Answer from the drawing. Dimensions are ordinates in mm from the lowest x, y and z of the part. A direction names the side the tool comes from. Coordinates: 2 decimals unless noted, no trailing zeros. Order: outer loops, then holes, each group sorted by start corner. A loop starts at its lowest first (then second) coordinate and runs counter-clockwise, first axis right, second up.
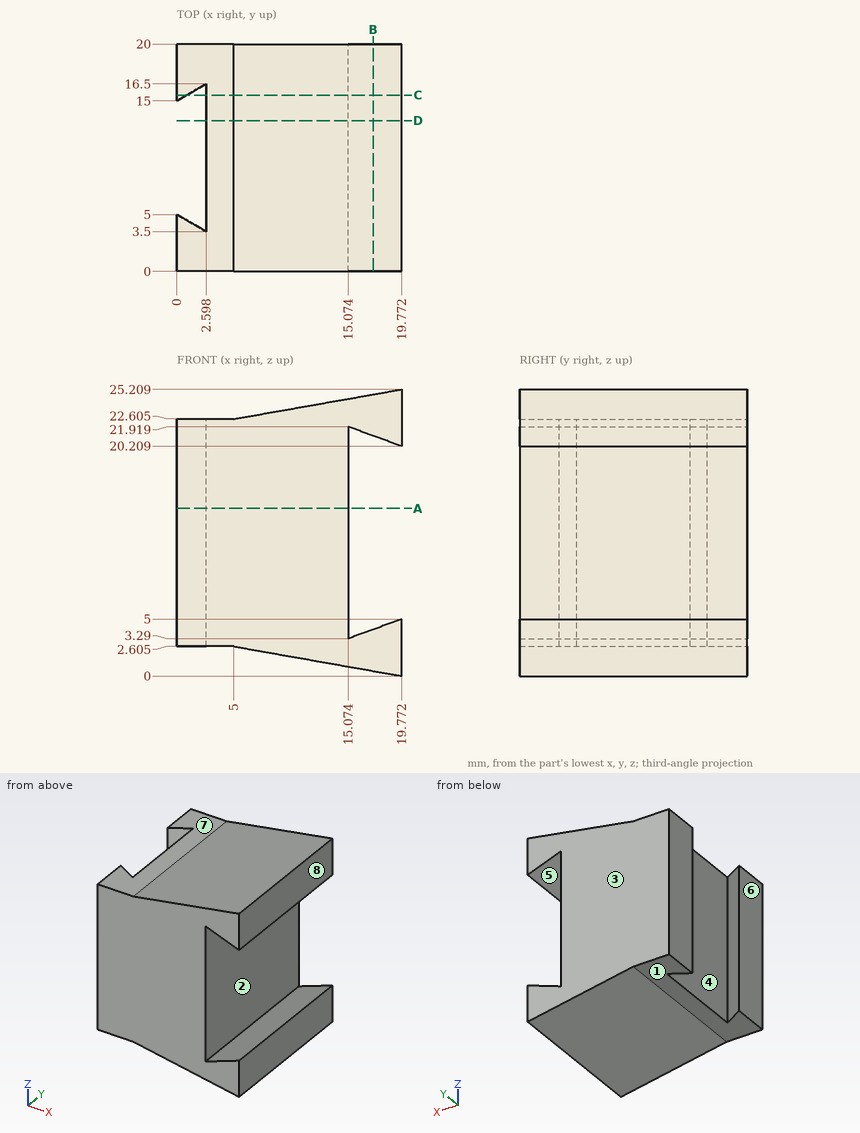
1) Consider L1, parallel to Z at x = 1.5, y = 1.5 (1 decimal); L2, parallel to X at y = 8.75, z = 6.75; L3, parallel to Z at x = 16.5, y = 3.25. Determine where each line is inside the solid, lowest interval first.
2) Section B-B (x = 17.25) is taken. Give the vertices of the cut face in (y, z) (1 decimal).
3) Section A-A (z = 14.75) is taken. Give the vertices of the cut face in (x, y).
4) Section C-C (y = 15.5) is taken. Give the vertices of the cut face in (x, z) (1 decimal).
5) Section D-D (y = 13.25) is taken. Give the vertices of the cut face in (x, z) (1 decimal).
6) A tool of negligible diameter and unlimited length cuts with its end or side. For the marked faces 4, 5, 6, 7 and 8, from which of +Z, -Z, +X, -X, +Y, -Y can it reach the whole face along a straight path? Write none if from no direction.
7) Each of these flat-tipped pins is pushed along its axis until it touches: P1, Ø3, axis at y = 12.5, z = 6, coming from the -X side; P2, Ø1.5, axis at x = 3.5, y = 15, coming from the -Z side (1 decimal); P3, Ø5, axis at y = 7.5, z = 10, coming from the +X side. Where does it stop, or does it pass through?
8) Determine the mould class of the marked faces 1, 2 and 3 for opening direction Z: released by +Z, released by -Z, zero draft, split by the parting line, or undercut.
Filled sheet:
1. L1: z = 2.6 to 22.6
1. L2: x = 2.6 to 15.07
1. L3: z = 0.58 to 3.81, 21.4 to 24.63
2. outline: (0, 0.4) - (20, 0.4) - (20, 4.1) - (0, 4.1) - close; (0, 21.1) - (20, 21.1) - (20, 24.8) - (0, 24.8) - close
3. outline: (0, 0) - (15.07, 0) - (15.07, 20) - (0, 20) - (0, 15) - (2.6, 16.5) - (2.6, 3.5) - (0, 5) - close
4. outline: (0, 2.6) - (0.9, 2.6) - (0.9, 22.6) - (0, 22.6) - close; (2.6, 2.6) - (5, 2.6) - (19.8, 0) - (19.8, 5) - (15.1, 3.3) - (15.1, 21.9) - (19.8, 20.2) - (19.8, 25.2) - (5, 22.6) - (2.6, 22.6) - close
5. outline: (2.6, 2.6) - (5, 2.6) - (19.8, 0) - (19.8, 5) - (15.1, 3.3) - (15.1, 21.9) - (19.8, 20.2) - (19.8, 25.2) - (5, 22.6) - (2.6, 22.6) - close
6. face 4: +Z, -Z
6. face 5: +Y, -Y
6. face 6: +Z, -Z, -X, +Y, -Y
6. face 7: +Z, -X, +Y, -Y
6. face 8: +Z, -Z, +X, +Y, -Y
7. P1: stops at x = 2.6
7. P2: stops at z = 2.6
7. P3: stops at x = 15.07
8. face 1: released by -Z
8. face 2: undercut
8. face 3: zero draft
